Geometry check sheet. Reference: drawing and pictorial views, mm from the part's lowest x, y, z. Round coordinates to 2 decimals unless told otherwise and drop trailing zeros. Order: outer loops, then holes, each group sorted by start corner. A loop starts at its lowest first (then second) coordinate and runs counter-clockwise, first axis right, second up.
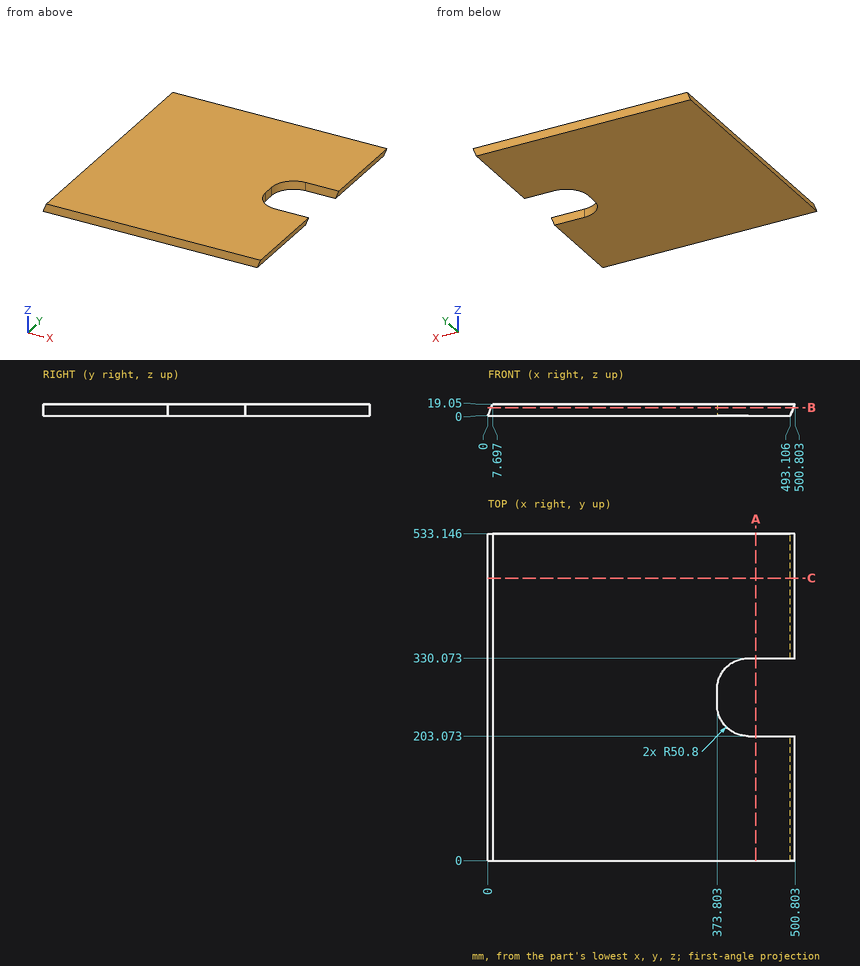
1) Sectioned sample at B-B on z = 13. Record the cut outline in (x, y).
2) Scan lines: probe 1 along Y at (x, z) = (463.5, 3); probe 2 along Y at (x, z) = (422.5, 11); probe 3 along X at (y, z) = (373.5, 15.25). Record each from-to range of solid material in increasing order.
3) Sectioned sample at A-A on x = 437. Record the cut outline in (y, z), then the cut area to 3 significant figures.
4) Sectioned sample at C-C on y = 460.5. Record the cut outline in (x, z), then the cut area to 3 significant figures.
5) Go/stop test with flat-tipped pins: pin 1 Ø2 at (y, z) = (121.5, 16) entering from +X (1 decimal); pin 2 Ø8 at (y, z) = (373, 15) entering from +X; pin 3 Ø10 at (y, z) = (207.5, 15.5) entering from +X. Record where each tip stops, or that it passes through.
Returned:
1. outline: (5.25, 0) - (498.36, 0) - (498.36, 203.07) - (424.6, 203.07) arc R50.8 cw to (373.8, 253.87) - (373.8, 279.27) arc R50.8 cw to (424.6, 330.07) - (498.36, 330.07) - (498.36, 533.15) - (5.25, 533.15) - close
2. probe 1: y = 0 to 203.07, 330.07 to 533.15
2. probe 2: y = 0 to 203.12, 330.03 to 533.15
2. probe 3: x = 6.16 to 499.27
3. outline: (0, 0) - (203.07, 0) - (203.07, 19.05) - (0, 19.05) - close; (330.07, 0) - (533.15, 0) - (533.15, 19.05) - (330.07, 19.05) - close
3. area: 7,740 mm2
4. outline: (0, 0) - (493.11, 0) - (500.8, 19.05) - (7.7, 19.05) - close
4. area: 9,390 mm2
5. pin 1: stops at x = 500
5. pin 2: stops at x = 500.78
5. pin 3: stops at x = 500.31
